```python
from build123d import *

# Parameters (mm, degrees)
BOSS_EXTRUDE1_DEPTH     = 15
CUT_EXTRUDE1_DEPTH      = 41.397648446
CUT_EXTRUDE1_DEPTH_BACK = 41.397648446
FILLET1_R               = 0.4
FILLET2_R               = 0.5
CUT_EXTRUDE2_REACH      = 40.314
SKETCH3_R               = 4.25
CUT_EXTRUDE3_DEPTH      = 12.9
SKETCH6_W               = 11
SKETCH6_H               = 48
CUT_EXTRUDE4_DEPTH      = 1
FILLET3_R               = 5
CHAMFER1_SIZE           = 0.5
BOSS_EXTRUDE2_DEPTH     = 2
CUT_EXTRUDE5_DEPTH      = 24
CUT_EXTRUDE5_DEPTH_BACK = 24
CUT_EXTRUDE6_DEPTH      = 0.5


with BuildPart() as part:
    # Sketch1 → Boss-Extrude1 (new, symmetric)
    with BuildSketch(Plane(origin=(0, 0, 0), x_dir=(0, 0, -1), z_dir=(1, 0, 0))):
        Polygon((32.4, -8.973205081), (32.4, 0), (-32.4, 0), (-32.4, -8.973205081), (-29.4977786, -14), (-32.326794919, -18.9), (32.326794919, -18.9), (29.4977786, -14), align=None)
    extrude(amount=BOSS_EXTRUDE1_DEPTH, both=True)

    # Sketch2 → Cut-Extrude1 (cut, two sides: drawn at the far end of the back side and taken through both)
    with BuildSketch(Plane.XY.offset(-CUT_EXTRUDE1_DEPTH_BACK)):
        Polygon((8.943375673, -5), (-8.943375673, -5), (-6.056624327, 0), (0, 0), (6.056624327, 0), align=None)
    extrude(amount=CUT_EXTRUDE1_DEPTH + CUT_EXTRUDE1_DEPTH_BACK, mode=Mode.SUBTRACT)

    # Fillet1
    fillet1_edges = [part.edges().sort_by_distance(p)[0] for p in [
        (0, -18.9, -32.326794919),
        (0, -18.9, 32.326794919),
        (0, -8.973205081, 32.4),
        (0, -8.973205081, -32.4),
        (6.056624327, 0, 0),
        (-6.056624327, 0, 0),
    ]]
    fillet(fillet1_edges, radius=FILLET1_R)

    # Fillet2
    fillet2_edges = [part.edges().sort_by_distance(p)[0] for p in [
        (0, -14, -29.4977786),
        (0, -14, 29.4977786),
        (8.943375673, -5, 0),
        (-8.943375673, -5, 0),
    ]]
    fillet(fillet2_edges, radius=FILLET2_R)

    # Sketch3 → Cut-Extrude2 (cut, up to next)
    with BuildSketch(Plane(origin=(0, -5, 0), x_dir=(1, 0, 0), z_dir=(0, 1, 0)), mode=Mode.PRIVATE) as cut_extrude2_sk1:
        with Locations(Location((0, 18, 0), (0, 0, 270))):
            Circle(SKETCH3_R)
    cut_extrude2_tool1 = extrude(cut_extrude2_sk1.sketch, amount=-CUT_EXTRUDE2_REACH, mode=Mode.PRIVATE) & part.part
    # Sketch3 → Cut-Extrude2 (cut, up to next)
    with BuildSketch(Plane(origin=(0, -5, 0), x_dir=(1, 0, 0), z_dir=(0, 1, 0)), mode=Mode.PRIVATE) as cut_extrude2_sk2:
        with Locations(Location((0, -18, 0), (0, 0, 270))):
            Circle(SKETCH3_R)
    cut_extrude2_tool2 = extrude(cut_extrude2_sk2.sketch, amount=-CUT_EXTRUDE2_REACH, mode=Mode.PRIVATE) & part.part
    # Sketch3 → Cut-Extrude2 (cut, up to next)
    with BuildSketch(Plane(origin=(0, -5, 0), x_dir=(1, 0, 0), z_dir=(0, 1, 0)), mode=Mode.PRIVATE) as cut_extrude2_sk3:
        with Locations(Location((0, 6, 0), (0, 0, 270))):
            Circle(SKETCH3_R)
    cut_extrude2_tool3 = extrude(cut_extrude2_sk3.sketch, amount=-CUT_EXTRUDE2_REACH, mode=Mode.PRIVATE) & part.part
    # Sketch3 → Cut-Extrude2 (cut, up to next)
    with BuildSketch(Plane(origin=(0, -5, 0), x_dir=(1, 0, 0), z_dir=(0, 1, 0)), mode=Mode.PRIVATE) as cut_extrude2_sk4:
        with Locations(Location((0, -6, 0), (0, 0, 270))):
            Circle(SKETCH3_R)
    cut_extrude2_tool4 = extrude(cut_extrude2_sk4.sketch, amount=-CUT_EXTRUDE2_REACH, mode=Mode.PRIVATE) & part.part
    add(cut_extrude2_tool1.solids().sort_by_distance((0, -5, -18))[0], mode=Mode.SUBTRACT)
    add(cut_extrude2_tool2.solids().sort_by_distance((0, -5, 18))[0], mode=Mode.SUBTRACT)
    add(cut_extrude2_tool3.solids().sort_by_distance((0, -5, -6))[0], mode=Mode.SUBTRACT)
    add(cut_extrude2_tool4.solids().sort_by_distance((0, -5, 6))[0], mode=Mode.SUBTRACT)

    # Sketch5 → Cut-Extrude3 (cut)
    with BuildSketch(Plane(origin=(0, -5, 0), x_dir=(1, 0, 0), z_dir=(0, 1, 0))):
        Polygon((-2.828427125, 22.5254834), (4.5254834, 15.171572875), (2.828427125, 13.4745166), (-4.5254834, 20.828427125), align=None)
        Polygon((-2.828427125, 10.5254834), (4.5254834, 3.171572875), (2.828427125, 1.4745166), (-4.5254834, 8.828427125), align=None)
        Polygon((-2.828427125, -1.4745166), (4.5254834, -8.828427125), (2.828427125, -10.5254834), (-4.5254834, -3.171572875), align=None)
        Polygon((-2.828427125, -13.4745166), (4.5254834, -20.828427125), (2.828427125, -22.5254834), (-4.5254834, -15.171572875), align=None)
    extrude(amount=-CUT_EXTRUDE3_DEPTH, mode=Mode.SUBTRACT)

    # Sketch6 → Cut-Extrude4 (cut)
    with BuildSketch(Plane(origin=(0, -5, 0), x_dir=(1, 0, 0), z_dir=(0, 1, 0))):
        Rectangle(SKETCH6_W, SKETCH6_H)
    extrude(amount=-CUT_EXTRUDE4_DEPTH, mode=Mode.SUBTRACT)

    # Fillet3
    fillet3_edges = [part.edges().sort_by_distance(p)[0] for p in [
        (-5.5, -5.5, 24),
        (-5.5, -5.5, -24),
        (5.5, -5.5, -24),
        (5.5, -5.5, 24),
    ]]
    fillet(fillet3_edges, radius=FILLET3_R)

    # Chamfer1
    chamfer1_edges = [part.edges().sort_by_distance(p)[0] for p in [
        (0, -18.9, 13.75),
        (0, -18.9, -22.25),
        (0, -18.9, 1.75),
        (0, -18.9, -10.25),
    ]]
    chamfer(chamfer1_edges, length=CHAMFER1_SIZE)

    # Sketch8 → Boss-Extrude2 (add)
    with BuildSketch(Plane(origin=(15, 0, 0), x_dir=(0, 0, -1), z_dir=(1, 0, 0))):
        Polygon((-32.4, -8.866025404), (-32.4, -18.9), (-31.633974596, -18.9), (31.633974596, -18.9), (32.4, -18.9), (32.4, -8.866025404), (32.4, 0), (-32.4, 0), align=None)
    extrude(amount=-BOSS_EXTRUDE2_DEPTH)

    # Sketch9 → Cut-Extrude5 (cut, two sides: drawn at the far end of the back side and taken through both)
    with BuildSketch(Plane.XY.offset(-CUT_EXTRUDE5_DEPTH_BACK)):
        Polygon((-15, -18.9), (-9, -18.9), (-15, -12.9), align=None)
    extrude(amount=CUT_EXTRUDE5_DEPTH + CUT_EXTRUDE5_DEPTH_BACK, mode=Mode.SUBTRACT)

    # Sketch10 → Cut-Extrude6 (cut)
    with BuildSketch(Plane(origin=(0, 0, 0), x_dir=(1, 0, 0), z_dir=(0, 1, 0))):
        with BuildLine():
            Line((8.874722325, -5.25), (12.874722325, -5.25))
            ThreePointArc((12.874722325, -5.25), (13.624722325, -6), (12.874722325, -6.75))
            Line((12.874722325, -6.75), (8.874722325, -6.75))
            ThreePointArc((8.874722325, -6.75), (8.124722325, -6), (8.874722325, -5.25))
        make_face()
        with BuildLine():
            Line((8.874722325, 17.5), (12.874722325, 17.5))
            ThreePointArc((12.874722325, 17.5), (13.624722325, 16.75), (12.874722325, 16))
            Line((12.874722325, 16), (8.874722325, 16))
            ThreePointArc((8.874722325, 16), (8.124722325, 16.75), (8.874722325, 17.5))
        make_face()
        with BuildLine():
            Line((8.874722325, 20), (12.874722325, 20))
            ThreePointArc((12.874722325, 20), (13.624722325, 19.25), (12.874722325, 18.5))
            Line((12.874722325, 18.5), (8.874722325, 18.5))
            ThreePointArc((8.874722325, 18.5), (8.124722325, 19.25), (8.874722325, 20))
        make_face()
        with BuildLine():
            Line((8.874722325, -19.75), (12.874722325, -19.75))
            ThreePointArc((12.874722325, -19.75), (13.624722325, -20.5), (12.874722325, -21.25))
            Line((12.874722325, -21.25), (8.874722325, -21.25))
            ThreePointArc((8.874722325, -21.25), (8.124722325, -20.5), (8.874722325, -19.75))
        make_face()
        with BuildLine():
            Line((8.874722325, -17.25), (12.874722325, -17.25))
            ThreePointArc((12.874722325, -17.25), (13.624722325, -18), (12.874722325, -18.75))
            Line((12.874722325, -18.75), (8.874722325, -18.75))
            ThreePointArc((8.874722325, -18.75), (8.124722325, -18), (8.874722325, -17.25))
        make_face()
        with BuildLine():
            Line((8.874722325, -14.75), (12.874722325, -14.75))
            ThreePointArc((12.874722325, -14.75), (13.624722325, -15.5), (12.874722325, -16.25))
            Line((12.874722325, -16.25), (8.874722325, -16.25))
            ThreePointArc((8.874722325, -16.25), (8.124722325, -15.5), (8.874722325, -14.75))
        make_face()
        with BuildLine():
            Line((8.874722325, 5.5), (12.874722325, 5.5))
            ThreePointArc((12.874722325, 5.5), (13.624722325, 4.75), (12.874722325, 4))
            Line((12.874722325, 4), (8.874722325, 4))
            ThreePointArc((8.874722325, 4), (8.124722325, 4.75), (8.874722325, 5.5))
        make_face()
        with BuildLine():
            Line((8.874722325, 8), (12.874722325, 8))
            ThreePointArc((12.874722325, 8), (13.624722325, 7.25), (12.874722325, 6.5))
            Line((12.874722325, 6.5), (8.874722325, 6.5))
            ThreePointArc((8.874722325, 6.5), (8.124722325, 7.25), (8.874722325, 8))
        make_face()
        with BuildLine():
            Line((8.874722325, 10.5), (12.874722325, 10.5))
            ThreePointArc((12.874722325, 10.5), (13.624722325, 9.75), (12.874722325, 9))
            Line((12.874722325, 9), (8.874722325, 9))
            ThreePointArc((8.874722325, 9), (8.124722325, 9.75), (8.874722325, 10.5))
        make_face()
        with BuildLine():
            Line((8.874722325, 3), (12.874722325, 3))
            ThreePointArc((12.874722325, 3), (13.624722325, 2.25), (12.874722325, 1.5))
            Line((12.874722325, 1.5), (8.874722325, 1.5))
            ThreePointArc((8.874722325, 1.5), (8.124722325, 2.25), (8.874722325, 3))
        make_face()
    extrude(amount=-CUT_EXTRUDE6_DEPTH, mode=Mode.SUBTRACT)


solid = part.part
```
Can you work these out from the model? Positions are in its coordinate system, mm. A direction names the side the tool comes from. Round coordinates to 2 decimals unless told otherwise and drop trailing zeros. Order: outer loops, then holes, each group sorted by start corner. A loop starts at its lowest first (then second) coordinate and runs counter-clockwise, first axis right, second up.
(1) If we section it at A-A (y = -2.5): Please give me the cut outline in (x, z).
Results are:
outline: (-15, -32.4) - (-7.5, -32.4) - (-7.5, 32.4) - (-15, 32.4) - close; (7.5, -32.4) - (15, -32.4) - (15, 32.4) - (7.5, 32.4) - close
(2) If we section it at C-C (y = -7.5): Count the separate pieces of the cut face and the enclosed holes in it, plus the area to 3 significant figures.
Results are:
separate pieces: 1
enclosed holes: 4
area: 1,700 mm2
(3) We'd pull the mould along X, two halves only. Please class faces 6 (the face through (-12, -15.9, -0.3)), 7 (the face through (-3.689, -11.867, -21.665)), 8 (the face through (-0.804, -16.247, 30.795)): +X half, -X half, draft (parallel to the pull), parting line (faces both ways), or undercut.
Results are:
face 6: -X half
face 7: undercut
face 8: draft
(4) If we section it at B-B (z = 6): Please give me the cut outline in (x, y), plus the area to 3 significant figures.
Results are:
outline: (-15, -12.9) - (-9, -18.9) - (-4.75, -18.9) - (-4.25, -18.4) - (-4.25, -6) - (-5.5, -6) - (-5.5, -5) - (-8.08, -5) arc R0.5 cw to (-8.51, -4.25) - (-6.4, -0.6) arc R0.4 ccw to (-6.75, 0) - (-15, 0) - close; (4.25, -18.4) - (4.75, -18.9) - (15, -18.9) - (15, 0) - (13.62, 0) - (13.62, -0.5) - (8.12, -0.5) - (8.12, 0) - (6.75, 0) arc R0.4 ccw to (6.4, -0.6) - (8.51, -4.25) arc R0.5 cw to (8.08, -5) - (5.5, -5) - (5.5, -6) - (4.25, -6) - close
area: 350 mm2
(5) On a 3-axis mill with a long thin cutter (end or side, diameter ignored), from which of +Z, -Z, +X, -X, +Y, -Y can I reach the whole of each face in a straight line? I mean faces 1 (the face through (-15, -7, 0)), 2 (the face through (-13, -17, 24)), 3 (the face through (-0.804, -16.303, -30.828)), 4 (the face through (3.689, -11.867, 9.665)), 5 (the face through (11, 0, 0)). Say none if no direction works.
Results are:
face 1: +Z, -Z, -X, +Y, -Y
face 2: -X, -Y
face 3: -Z, -X
face 4: +Y
face 5: +Z, -Z, +X, -X, +Y
(6) If I drill on L1, parallel to Z at x = 0, y = -14; L2, parallel to Z at x = 0, y = -8.5; L3, parallel to X at y = -10, z = 6, over which ranges is the centre line in solid material (lowest first)?
Results are:
L1: z = -29.58 to -22.25, -13.75 to -10.25, -1.75 to 1.75, 10.25 to 13.75, 22.25 to 29.58
L2: z = -32.4 to -22.25, -13.75 to -10.25, -1.75 to 1.75, 10.25 to 13.75, 22.25 to 32.4
L3: x = -15 to -4.25, 4.25 to 15
(7) I'm going to push flat-ended pins straight in: pin 1 (4 mm diameter, centred on x = -9.5, y = -11.5, fed in from +Z); pin 2 (2.5 mm diameter, centred on x = -2.5, z = -21, fed in from +Y); pin 3 (0.8 mm diameter, centred on x = 11.5, z = -5, fed in from +Y). Where does each tip first touch, or does it pass through?
Results are:
pin 1: stops at z = 32.1
pin 2: stops at y = -6
pin 3: stops at y = -0.5
